from build123d import *

# Parameters (mm, degrees)
F0_W = 2
F0_H = 70
F2_R = 0.99999


# Not quite as in the source:
# - a fillet or chamfer is up to 0.001 mm smaller than in the source, because OpenCascade refuses the exact size


with BuildPart() as f1:
    # F0 (on Front) → F1 (revolve)
    with BuildSketch(Plane.XZ):
        with Locations((-7.899047263, 13.5642557819)):
            Rectangle(F0_W, F0_H)
    revolve(axis=Axis((11.100952737, 0, 13.5642557819), (0, 0, -1)))

    # F2 (radius 1 in the source; OpenCascade refuses exactly that, so slightly less here)
    f2_edges = [f1.edges().sort_by_distance(p)[0] for p in [
        (29.100953, 0, 48.564256),
        (31.100953, 0, 48.564256),
        (31.100953, 0, -21.435744),
        (29.100953, 0, -21.435744),
    ]]
    fillet(f2_edges, radius=F2_R)


solid = f1.part
Source: CAD feature listing. Evaluate the final solid. Frame: model axes, mm. Coordinates: 2 decimals unless noted, no trailing zeros. Loops run counter-clockwise (first coordinate to the right, second up) from the corner with the lowest first, then second, coordinate; pieces in that order, holes last. Notation, with made-up numbers: (89, 17.5) - (114, 17.5) arc R16 ccw to (114, 48.5) - close; hole circle Ø10 at (56, 64). An arc over 180 degrees is marked (long way). One line per item, written item: value. Start each with the question number.
1. Ray query, L1, parallel to Y at x = 7, z = -15.5; L2, parallel to X at y = -16.5, z = -10; L3, parallel to X at y = -14, z = 43. Return the intervals inside material, ascending.
2. Section B-B (z = 5). Return the cut outline in (x, y).
3. Contact query for flat-ended pins moving along their axis: P1, Ø1.5, axis at x = 22, z = 18, coming from the +Y side; P2, Ø1.5, axis at x = 21.5, z = 27.5, coming from the -Y side; P3, Ø6, axis at x = 8.5, z = -2, coming from the -Y side. Output: stop coordinate, or through.
4. Mould query, pull axis X, two halves, no side actions, for faces 1 (the cylindrical face through (-7.374, -7.66, 14.04)), 2 (the cylindrical face through (-6.068, 5.407, 14.04)). Classes: pulls with the +X half, pulls with the -X half, needs draft (parallel to the pull), parting line crosses it, or undercut.
Verdict:
1. L1: y = -19.58 to -17.53, 17.53 to 19.58
1. L2: x = -0.2 to 3.91, 18.29 to 22.4
1. L3: x = -3.18 to -0.21, 22.41 to 25.38
2. outline: circle Ø40 at (11.1, 0); hole circle Ø36 at (11.1, 0)
3. P1: stops at y = 17.23
3. P2: stops at y = -17.52
3. P3: stops at y = -20
4. face 1: parting line crosses it
4. face 2: undercut
